```python
from build123d import *

# Parameters (mm, degrees)
ESQUISSE1_R        = 1.5
BOSS_EXTRU_2_DEPTH = 5


with BuildPart() as part:
    # Esquisse1 → Boss.-Extru.2 (new body)
    # profile 1 of 10: a face of its own
    with BuildSketch(Plane.XY):
        with BuildLine():
            ThreePointArc((-40, 0), (0, 40), (40, 0))
            Line((40, 0), (45, 0))
            ThreePointArc((45, 0), (42.690748412, 14.230249471), (36, 27))
            ThreePointArc((36, 27), (31.819805153, 31.819805153), (27, 36))
            ThreePointArc((27, 36), (0, 45), (-27, 36))
            ThreePointArc((-27, 36), (-31.819805153, 31.819805153), (-36, 27))
            ThreePointArc((-36, 27), (-42.690748412, 14.230249471), (-45, 0))
            Line((-45, 0), (-40, 0))
        make_face()
    # profile 2 of 10: a face of its own
    with BuildSketch(Plane.XY):
        with BuildLine():
            Line((45, 0), (40, 0))
            ThreePointArc((40, 0), (0, -40), (-40, 0))
            Line((-40, 0), (-45, 0))
            ThreePointArc((-45, 0), (-42.690748412, -14.230249471), (-36, -27))
            ThreePointArc((-36, -27), (-31.819805153, -31.819805153), (-27, -36))
            ThreePointArc((-27, -36), (0, -45), (27, -36))
            ThreePointArc((27, -36), (31.819805153, -31.819805153), (36, -27))
            ThreePointArc((36, -27), (42.690748412, -14.230249471), (45, 0))
        make_face()
    # profile 3 of 10: a face of its own
    with BuildSketch(Plane.XY):
        with BuildLine():
            ThreePointArc((-40, 0), (0, 40), (40, 0))
            Line((40, 0), (45, 0))
            ThreePointArc((45, 0), (42.690748412, 14.230249471), (36, 27))
            ThreePointArc((36, 27), (31.819805153, 31.819805153), (27, 36))
            ThreePointArc((27, 36), (0, 45), (-27, 36))
            ThreePointArc((-27, 36), (-31.819805153, 31.819805153), (-36, 27))
            ThreePointArc((-36, 27), (-42.690748412, 14.230249471), (-45, 0))
            Line((-45, 0), (-40, 0))
        make_face()
    # profile 4 of 10: a face of its own
    with BuildSketch(Plane.XY):
        with BuildLine():
            Line((45, 0), (40, 0))
            ThreePointArc((40, 0), (0, -40), (-40, 0))
            Line((-40, 0), (-45, 0))
            ThreePointArc((-45, 0), (-42.690748412, -14.230249471), (-36, -27))
            ThreePointArc((-36, -27), (-31.819805153, -31.819805153), (-27, -36))
            ThreePointArc((-27, -36), (0, -45), (27, -36))
            ThreePointArc((27, -36), (31.819805153, -31.819805153), (36, -27))
            ThreePointArc((36, -27), (42.690748412, -14.230249471), (45, 0))
        make_face()
    # profile 5 of 10: a face of its own
    with BuildSketch(Plane.XY):
        with BuildLine():
            ThreePointArc((-27, 36), (0, 45), (27, 36))
            Line((27, 36), (3, 54))
            ThreePointArc((3, 54), (0, 55), (-3, 54))
            Line((-3, 54), (-27, 36))
        make_face()
        with Locations((0, 50)):
            Circle(ESQUISSE1_R, mode=Mode.SUBTRACT)
    # profile 6 of 10: a face of its own
    with BuildSketch(Plane.XY):
        with BuildLine():
            Line((48.5, 0), (45, 0))
            ThreePointArc((45, 0), (42.690748412, -14.230249471), (36, -27))
            Line((36, -27), (54, -3))
            ThreePointArc((54, -3), (54.74341649, -1.58113883), (55, 0))
            Line((55, 0), (51.5, 0))
            ThreePointArc((51.5, 0), (50, -1.5), (48.5, 0))
        make_face()
    # profile 7 of 10: a face of its own
    with BuildSketch(Plane.XY):
        with BuildLine():
            ThreePointArc((36, 27), (42.690748412, 14.230249471), (45, 0))
            Line((45, 0), (48.5, 0))
            ThreePointArc((48.5, 0), (50, 1.5), (51.5, 0))
            Line((51.5, 0), (55, 0))
            ThreePointArc((55, 0), (54.74341649, 1.58113883), (54, 3))
            Line((54, 3), (36, 27))
        make_face()
    # profile 8 of 10: a face of its own
    with BuildSketch(Plane.XY):
        with BuildLine():
            Line((3, -54), (27, -36))
            ThreePointArc((27, -36), (0, -45), (-27, -36))
            Line((-27, -36), (-3, -54))
            ThreePointArc((-3, -54), (0, -55), (3, -54))
        make_face()
        with Locations((0, -50)):
            Circle(ESQUISSE1_R, mode=Mode.SUBTRACT)
    # profile 9 of 10: a face of its own
    with BuildSketch(Plane.XY):
        with BuildLine():
            Line((-48.5, 0), (-45, 0))
            ThreePointArc((-45, 0), (-42.690748412, 14.230249471), (-36, 27))
            Line((-36, 27), (-54, 3))
            ThreePointArc((-54, 3), (-54.74341649, 1.58113883), (-55, 0))
            Line((-55, 0), (-51.5, 0))
            ThreePointArc((-51.5, 0), (-50, 1.5), (-48.5, 0))
        make_face()
    # profile 10 of 10: a face of its own
    with BuildSketch(Plane.XY):
        with BuildLine():
            ThreePointArc((-36, -27), (-42.690748412, -14.230249471), (-45, 0))
            Line((-45, 0), (-48.5, 0))
            ThreePointArc((-48.5, 0), (-50, -1.5), (-51.5, 0))
            Line((-51.5, 0), (-55, 0))
            ThreePointArc((-55, 0), (-54.74341649, -1.58113883), (-54, -3))
            Line((-54, -3), (-36, -27))
        make_face()
    extrude(amount=BOSS_EXTRU_2_DEPTH)


solid = part.part
```
The model under review builds one solid part; all positions refer to its coordinate system, in mm. Round coordinates to 2 decimals unless told otherwise and drop trailing zeros. Loops run counter-clockwise (first coordinate to the right, second up) from the corner with the lowest first, then second, coordinate; pieces in that order, holes last. Notation, with made-up numbers: (50, 6.25) -> (72, 6.25) arc R28 ccw to (72, 25.25) -> close; hole circle Ø4 at (76.5, 54.5). An arc over 180 degrees is marked (long way). Answer in a Markdown table with one row per item.
1) Wall thickness on line 1 along Y through (x, z) = (0, 2.1); line 2 along X through (y, z) = (37, 3.35); line 3 along X through (y, z) = (2, 4.05): over which ranges is each line inside the solid? List them lowest first.
Taken from the geometry:
| item | result |
|---|---|
| line 1 | y = -55 to -51.5, -48.5 to -40, 40 to 48.5, 51.5 to 55 |
| line 2 | x = -25.67 to -15.2, 15.2 to 25.67 |
| line 3 | x = -54.58 to -39.95, 39.95 to 54.58 |
2) Consider section C-C, the plane x = 50. Write out the cut boundary in (y, z), plus the area to 3 significant figures.
Taken from the geometry:
| item | result |
|---|---|
| outline | (-8.33, 0) -> (-1.5, 0) -> (-1.5, 5) -> (-8.33, 5) -> close; (1.5, 0) -> (8.33, 0) -> (8.33, 5) -> (1.5, 5) -> close |
| area | 68.3 mm² |
3) Consider section B-B, the plane z = 3.35. Write out the cut boundary in (x, y).
Taken from the geometry:
| item | result |
|---|---|
| outline | (-54, -3) -> (-36, -27) arc R45 ccw to (-27, -36) -> (-3, -54) arc R5 ccw to (3, -54) -> (27, -36) arc R45 ccw to (36, -27) -> (54, -3) arc R5 ccw to (54, 3) -> (36, 27) arc R45 ccw to (27, 36) -> (3, 54) arc R5 ccw to (-3, 54) -> (-27, 36) arc R45 ccw to (-36, 27) -> (-54, 3) arc R5 ccw to start; hole circle Ø3 at (-50, 0); hole circle Ø80 at (0, 0); hole circle Ø3 at (0, -50); hole circle Ø3 at (0, 50); hole circle Ø3 at (50, 0) |
4) For pin 1 Ø3 at (y, z) = (-21, 3.5) entering from +X (3 decimals); pin 2 Ø1 at (y, z) = (3.5, 2) entering from +X; pin 3 Ø1 at (y, z) = (-32.5, 1.5) entering from -X, all flat-tipped, find the tip position at first contact; note any pin that passes through.
Taken from the geometry:
| item | result |
|---|---|
| pin 1 | stops at x = 41.625 |
| pin 2 | stops at x = 54 |
| pin 3 | stops at x = -31.64 |
5) Consider section A-A, the plane x = 0. Write out the cut boundary in (y, z), plus the area to 3 significant figures.
Taken from the geometry:
| item | result |
|---|---|
| outline | (-55, 0) -> (-51.5, 0) -> (-51.5, 5) -> (-55, 5) -> close; (-48.5, 0) -> (-40, 0) -> (-40, 5) -> (-48.5, 5) -> close; (40, 0) -> (48.5, 0) -> (48.5, 5) -> (40, 5) -> close; (51.5, 0) -> (55, 0) -> (55, 5) -> (51.5, 5) -> close |
| area | 120 mm² |
6) Draft analysis for pull direction X (two halves, no side actions). For faces 1 (the cylindrical face through (-0.325, -51.464, 2.465)), 2 (the cylindrical face through (-31.88, -31.76, 2.46)), 3 (the cylindrical face through (-51.5, -0.07, 2.46)), 4 (the flat face through (45, -15, 2)), state which applies: pulls with the +X half, pulls with the -X half, needs draft (parallel to the pull), parting line crosses it, or undercut.
Taken from the geometry:
| item | result |
|---|---|
| face 1 | undercut |
| face 2 | pulls with the -X half |
| face 3 | undercut |
| face 4 | pulls with the +X half |
